Here's how the part is built. I have some questions about the finished solid (model axes, mm). Face numbers are marked on the shaded views. A direction names the side the tool comes from. Give positions to 0.01 mm unless a question says otherwise; leave off trailing zeros. Order: outer loops, then holes, each group sorted by start corner. A loop starts at its lowest first (then second) coordinate and runs counter-clockwise, first axis right, second up. Notation, with made-up numbers: (-22.75, 7.25) -> (-18.75, 7.25) arc R36 ccw to (-18.75, 44.25) -> close; hole circle Ø9 at (28, 11.5). An arc over 180 degrees is marked (long way). Write each question's results on one line, items separated by ' | '. Start each with the question number.
Q1. Imagine slicing it at D-D, the plane x = 28. Please give me the cut outline in (y, z), then the cut area to 3 significant figures.
Q2. I need wall thicknesses on line 1 along Z through (x, y) = (17, 1.5); line 2 along Z through (x, y) = (17, 14.7); line 3 along X through (y, z) = (14, -15). Which ranges of each line are inside material? Lowest first, please. Write a range as [from, to].
Q3. Imagine slicing it at B-B, the plane y = 34. Please give me the cut outline in (x, z).
Q4. For the marked faces 1, 2 and 3, which set-ups out of +Z, -Z, +X, -X, +Y, -Y let a thin tool reach every point of the face, with its end or its side?
Q5. I'm going to push flat-ended pins straight in: pin 1 (5 mm diameter, centred on x = 6, y = 23.5, fed in from +Z); pin 2 (4 mm diameter, centred on x = 19, z = 10.5, fed in from +Y); pin 3 (2.5 mm diameter, centred on x = 17, z = 14, fed in from +Y); pin 4 (5 mm diameter, centred on x = 29, z = -3, fed in from +Y). Where does each tip first touch, or does it pass through?
Q6. Imagine slicing it at A-A, the plane z = -15. Please give me the cut outline in (x, y).
Q7. Imagine slicing it at C-C, the plane x = 17. Please give me the cut outline in (y, z).
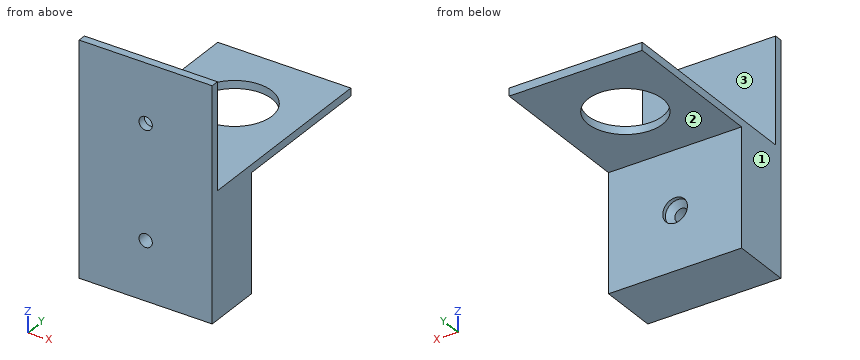
```python
from build123d import *

# Parameters (mm, degrees)
SKETCH1_W                                      = 34
SKETCH1_H                                      = 53
BOSS_EXTRUDE1_DEPTH                            = 2
SKETCH2_W                                      = 34
SKETCH2_H                                      = 2
BOSS_EXTRUDE2_DEPTH                            = 27
SKETCH3_W                                      = 34
SKETCH3_H                                      = 15
BOSS_EXTRUDE3_DEPTH                            = 30
SKETCH4_R                                      = 9.5
CUT_EXTRUDE1_DEPTH                             = 71.632853546
CSK_FOR_M3_FLAT_HEAD_MACHINE_SCREW1_AT_2_COUNT = 2
CSK_FOR_M3_FLAT_HEAD_MACHINE_SCREW1_AT_2_PITCH = 29


with BuildPart() as part:
    # Sketch1 → Boss-Extrude1 (new body)
    with BuildSketch(Plane.XY):
        with Locations((17, 26.5)):
            Rectangle(SKETCH1_W, SKETCH1_H)
    extrude(amount=BOSS_EXTRUDE1_DEPTH)

    # Sketch2 → Boss-Extrude2 (add)
    with BuildSketch(Plane.XY.offset(2)):
        with Locations((17, 1)):
            Rectangle(SKETCH2_W, SKETCH2_H)
    extrude(amount=BOSS_EXTRUDE2_DEPTH)

    # Sketch3 → Boss-Extrude3 (add)
    with BuildSketch(Plane(origin=(0, 0, 0), x_dir=(-1, 0, 0), z_dir=(0, 0, -1))):
        with Locations((-17, 7.5)):
            Rectangle(SKETCH3_W, SKETCH3_H)
    extrude(amount=BOSS_EXTRUDE3_DEPTH)

    # Sketch4 → Cut-Extrude1 (cut, through all)
    with BuildSketch(Plane.XY.offset(2)):
        with Locations((17, 34)):
            Circle(SKETCH4_R)
    extrude(amount=-CUT_EXTRUDE1_DEPTH, mode=Mode.SUBTRACT)

    # Sketch9 → CSK for M3 Flat Head Machine Screw1 (revolve, cut)
    with BuildSketch(Plane(origin=(17, 15, -15), x_dir=(0, 0, 1), z_dir=(1, 0, 0))):
        Polygon((0, 0), (0, 15), (1.7, 15), (1.7, 2.45), (3.15, 1), (3.15, 0), align=None)
    csk_for_m3_flat_head_machine_screw1 = revolve(axis=Axis((17, 21.35, -15), (0, -1, 0)), mode=Mode.SUBTRACT)

    # CSK for M3 Flat Head Machine Screw1 at 2: CSK for M3 Flat Head Machine Screw1 ×2
    with Locations(*[(0, 0, i * CSK_FOR_M3_FLAT_HEAD_MACHINE_SCREW1_AT_2_PITCH) for i in range(1, CSK_FOR_M3_FLAT_HEAD_MACHINE_SCREW1_AT_2_COUNT)]):
        add(csk_for_m3_flat_head_machine_screw1, mode=Mode.SUBTRACT)


solid = part.part
```
Geometry check:
1) outline: (0, -30) -> (15, -30) -> (15, 0) -> (53, 0) -> (53, 2) -> (2, 2) -> (2, 29) -> (0, 29) -> close | area: 610 mm²
2) line 1: [-30, -16.7], [-13.3, 12.3], [15.7, 29] | line 2: [-30, -18.15], [-11.85, 2] | line 3: [0, 13.85], [20.15, 34]
3) outline: (0, 0) -> (7.5, 0) -> (7.5, 2) -> (0, 2) -> close; (26.5, 0) -> (34, 0) -> (34, 2) -> (26.5, 2) -> close
4) face 1: +Z, -Z, -X, +Y, -Y | face 2: -Z, +X, -X, +Y | face 3: +Z, +X, -X, +Y
5) pin 1: z = 2 | pin 2: y = 2 | pin 3: through | pin 4: y = 15
6) outline: (0, 0) -> (15.3, 0) -> (15.3, 12.55) -> (13.85, 14) -> (13.85, 15) -> (0, 15) -> close; (18.7, 0) -> (34, 0) -> (34, 15) -> (20.15, 15) -> (20.15, 14) -> (18.7, 12.55) -> close
7) outline: (0, -30) -> (15, -30) -> (15, -18.15) -> (14, -18.15) -> (12.55, -16.7) -> (0, -16.7) -> close; (0, -13.3) -> (12.55, -13.3) -> (14, -11.85) -> (15, -11.85) -> (15, 0) -> (24.5, 0) -> (24.5, 2) -> (2, 2) -> (2, 12.3) -> (0, 12.3) -> close; (0, 15.7) -> (2, 15.7) -> (2, 29) -> (0, 29) -> close; (43.5, 0) -> (53, 0) -> (53, 2) -> (43.5, 2) -> close
